```python
from build123d import *

# Parameters (mm, degrees)
F1_DEPTH = 25.4
F5_DEPTH = 12.7
F6_DEPTH = 25.4
F7_DEPTH = 12.7


with BuildPart() as f1:
    # F0 (on Top) → F1 (new body)
    with BuildSketch(Plane.XY):
        Polygon((12.7, 27.191021), (12.7, 0), (25.4, 0), (25.4, 27.191021), (38.1, 27.191021), (38.1, 58.941021), (0, 58.941021), (0, 27.191021), align=None)
    extrude(amount=F1_DEPTH)

    # F3 (on face) → F5 (cut)
    with BuildSketch(Plane.YZ.offset(38.1)):
        Polygon((27.191021, 25.4), (27.191021, 0), (39.891021, 25.4), align=None)
    extrude(amount=-F5_DEPTH, mode=Mode.SUBTRACT)

    # F2 (on face) → F6 (cut)
    with BuildSketch(Plane.YZ.offset(25.4)):
        Polygon((0, 25.4), (0, 0), (12.7, 25.4), align=None)
    extrude(amount=-F6_DEPTH, mode=Mode.SUBTRACT)

    # F4 (on face) → F7 (cut)
    with BuildSketch(Plane(origin=(0, 0, 0), x_dir=(0, -1, 0), z_dir=(-1, 0, 0))):
        Polygon((-27.191021, 25.4), (-39.891021, 25.4), (-27.191021, 0), align=None)
    extrude(amount=-F7_DEPTH, mode=Mode.SUBTRACT)


solid = f1.part
```
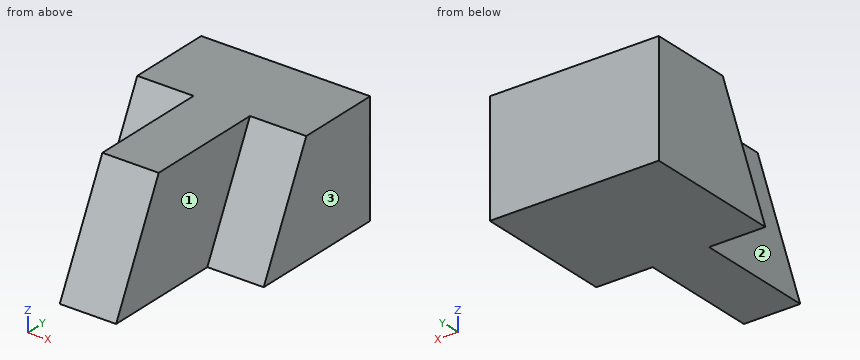
Could you check a few things on this model? Use its own coordinates, in mm. Face numbers are marked on the shaded views. A direction names the side the tool comes from. Coordinates: 2 decimals unless noted, no trailing zeros. Loops run counter-clockwise (first coordinate to the right, second up) from the corner with the lowest first, then second, coordinate; pieces in that order, holes last. Notation, with made-up numbers: M -19,-26.5 L -15,-26.5 A21 cw -15,-8.5 Z; hole C 69.5,0 d11. An arc over 180 degrees is marked long. Put each result on its own line as item: value. Start each with the question number.
(1) Suppose I cut it at C-C on y = 21. Please give me the cut outline in (x, z), then the cut area to 3 significant figures.
(2) Suppose I cut it at A-A on z = 4.75. Please give me the cut outline in (x, y) (3 decimals).
(3) I need wall thicknesses on line 1 (X direction, y = 6, z = 2.5); line 2 (Y direction, x = 29.5, z = 10); line 3 (Y direction, x = 34, z = 16.75). Which ranges of each line are inside material? Lowest first, please. Write a range as from..to.
(4) Suppose I cut it at D-D on z = 21.25. Please give me the cut outline in (x, y) (3 decimals), then the cut area to 3 significant figures.
(5) Suppose I cut it at B-B on x = 17.5. Please give me the cut outline in (y, z), then the cut area to 3 significant figures.
(6) For the marked faces 1, 2 and 3, which set-ups out of +Z, -Z, +X, -X, +Y, -Y let a thin tool reach every point of the face, with its end or its side?
(7) Will these pins go through, and if not, where does the flat tip stop? P1, Ø1.5, axis at y = 14, z = 14, coming from the -X side; P2, Ø2, axis at y = 23.5, z = 19, coming from the +X side; P3, Ø4, axis at x = 10.5, z = 8, coming from the -Y side.
Solutions:
1. outline: M 12.7,0 L 25.4,0 L 25.4,25.4 L 12.7,25.4 Z
1. area: 323 mm2
2. outline: M 0,29.566 L 12.7,29.566 L 12.7,2.375 L 25.4,2.375 L 25.4,29.566 L 38.1,29.566 L 38.1,58.941 L 0,58.941 Z
3. line 1: x = 12.7..25.4
3. line 2: y = 32.19..58.94
3. line 3: y = 35.57..58.94
4. outline: M 0,37.816 L 12.7,37.816 L 12.7,10.625 L 25.4,10.625 L 25.4,37.816 L 38.1,37.816 L 38.1,58.941 L 0,58.941 Z
4. area: 1,150 mm2
5. outline: M 0,0 L 58.94,0 L 58.94,25.4 L 12.7,25.4 Z
5. area: 1,340 mm2
6. face 1: +Z, +X, -Y
6. face 2: +Z, -X, -Y
6. face 3: +Z, -Z, +X, +Y, -Y
7. P1: stops at x = 12.7
7. P2: stops at x = 25.4
7. P3: stops at y = 30.19
